```python
from build123d import *

# Parameters (mm, degrees)
SKETCH1_W                = 82
SKETCH1_H                = 150
BOSS_EXTRUDE1_DEPTH      = 10
SKETCH2_W                = 10
SKETCH2_H                = 45
BOSS_EXTRUDE2_DEPTH      = 82
BOSS_EXTRUDE3_DEPTH      = 42
BOSS_EXTRUDE3_DEPTH_BACK = 10
FILLET3_RADIUS           = 26
FILLET3_LENGTH           = 10
FILLET4_RADIUS           = 26
FILLET4_LENGTH           = 10
BOSS_EXTRUDE4_DEPTH      = 10
BOSS_EXTRUDE5_DEPTH      = 10
FILLET5_R                = 15
FILLET6_R                = 15
SKETCH6_R                = 8
SKETCH6_R_2              = 5.5
CUT_EXTRUDE1_DEPTH       = 131.057679512
FILLET7_R                = 3
FILLET8_R                = 3
FILLET9_R                = 3
FILLET10_R               = 3
FILLET11_R               = 2
SKETCH7_R                = 5.5
CUT_EXTRUDE2_DEPTH       = 116.043470045
SKETCH8_W                = 188.706485039
SKETCH8_H                = 108.604028409
CUT_EXTRUDE3_DEPTH       = 126.678160394
SKETCH9_W                = 188.802330386
SKETCH9_H                = 115.284492933
CUT_EXTRUDE4_DEPTH       = 119.718153624
SKETCH10_W               = 24.217021772
SKETCH10_H               = 20.660675918
SKETCH10_W_2             = 13.71733401
SKETCH10_H_2             = 13.378634406
BOSS_EXTRUDE6_DEPTH      = 10


with BuildPart() as part:
    # Sketch1 → Boss-Extrude1 (new body)
    with BuildSketch(Plane(origin=(0, 0, 0), x_dir=(1, 0, 0), z_dir=(0, 1, 0))):
        Rectangle(SKETCH1_W, SKETCH1_H)
    extrude(amount=BOSS_EXTRUDE1_DEPTH)

    # Sketch2 → Boss-Extrude2 (add, through all)
    with BuildSketch(Plane(origin=(41, 0, 0), x_dir=(0, 0, -1), z_dir=(1, 0, 0))):
        with Locations((70, 22.5)):
            Rectangle(SKETCH2_W, SKETCH2_H)
    extrude(amount=-BOSS_EXTRUDE2_DEPTH)

    # Sketch3 → Boss-Extrude3 (add, two sides: drawn at the far end of the back side and taken through both)
    with BuildSketch(Plane.XY.offset(-65).offset(-BOSS_EXTRUDE3_DEPTH_BACK)):
        Polygon((10, 45), (10, 10), (20, 10), (20, 45), (20, 87), (10, 87), align=None)
        Polygon((-10, 45), (-10, 87), (-20, 87), (-20, 45), (-20, 10), (-10, 10), align=None)
    extrude(amount=BOSS_EXTRUDE3_DEPTH + BOSS_EXTRUDE3_DEPTH_BACK)

    # Fillet3: full round fillet: the end face becomes a half cylinder, R = half its width
    fillet3_face = Plane((15, 87, -49), x_dir=(-1, 0, 0), z_dir=(0, 1, 0))  # on the end face: x along it, z out of the body
    fillet3_slab = fillet3_face.offset(-FILLET3_RADIUS / 2) * Box(FILLET3_LENGTH, 2 * FILLET3_RADIUS, FILLET3_RADIUS, mode=Mode.PRIVATE)  # the body's end, R deep
    fillet3_round = Plane((15, 61, -49), x_dir=(0, 1, 0), z_dir=(-1, 0, 0)) * Cylinder(FILLET3_RADIUS, FILLET3_LENGTH, mode=Mode.PRIVATE)  # its axis R under the face
    add(fillet3_slab - fillet3_round, mode=Mode.SUBTRACT)

    # Fillet4: full round fillet: the end face becomes a half cylinder, R = half its width
    fillet4_face = Plane((-15, 87, -49), x_dir=(-1, 0, 0), z_dir=(0, 1, 0))  # on the end face: x along it, z out of the body
    fillet4_slab = fillet4_face.offset(-FILLET4_RADIUS / 2) * Box(FILLET4_LENGTH, 2 * FILLET4_RADIUS, FILLET4_RADIUS, mode=Mode.PRIVATE)  # the body's end, R deep
    fillet4_round = Plane((-15, 61, -49), x_dir=(0, 1, 0), z_dir=(-1, 0, 0)) * Cylinder(FILLET4_RADIUS, FILLET4_LENGTH, mode=Mode.PRIVATE)  # its axis R under the face
    add(fillet4_slab - fillet4_round, mode=Mode.SUBTRACT)

    # Sketch4 → Boss-Extrude4 (add)
    with BuildSketch(Plane(origin=(20, 0, 0), x_dir=(0, 0, -1), z_dir=(1, 0, 0))):
        Polygon((23, 10), (23, 50), (-75, 25), (-75, 10), align=None)
    extrude(amount=-BOSS_EXTRUDE4_DEPTH)

    # Sketch5 → Boss-Extrude5 (add)
    with BuildSketch(Plane.ZY.offset(20)):
        Polygon((-23, 50), (75, 25), (75, 10), (-23, 10), align=None)
    extrude(amount=-BOSS_EXTRUDE5_DEPTH)

    # Fillet5
    fillet5_edges = [part.edges().sort_by_distance(p)[0] for p in [
        (15, 25, 75),
    ]]
    fillet(fillet5_edges, radius=FILLET5_R)

    # Fillet6
    fillet6_edges = [part.edges().sort_by_distance(p)[0] for p in [
        (-15, 25, 75),
    ]]
    fillet(fillet6_edges, radius=FILLET6_R)

    # Sketch6 → Cut-Extrude1 (cut, through all)
    with BuildSketch(Plane(origin=(20, 0, 0), x_dir=(0, 0, -1), z_dir=(1, 0, 0))):
        with Locations((49, 61)):
            Circle(SKETCH6_R)
        with Locations((-60, 17.5)):
            Circle(SKETCH6_R_2)
    extrude(amount=-CUT_EXTRUDE1_DEPTH, mode=Mode.SUBTRACT)

    # Fillet7
    fillet7_edges = [part.edges().sort_by_distance(p)[0] for p in [
        (30.5, 45, -65),
    ]]
    fillet(fillet7_edges, radius=FILLET7_R)

    # Fillet8
    fillet8_edges = [part.edges().sort_by_distance(p)[0] for p in [
        (0, 45, -65),
    ]]
    fillet(fillet8_edges, radius=FILLET8_R)

    # Fillet9
    fillet9_edges = [part.edges().sort_by_distance(p)[0] for p in [
        (-30.5, 45, -65),
    ]]
    fillet(fillet9_edges, radius=FILLET9_R)

    # Fillet10
    fillet10_edges = [part.edges().sort_by_distance(p)[0] for p in [
        (30.5, 10, -65),
        (0, 10, -65),
        (-30.5, 10, -65),
    ]]
    fillet(fillet10_edges, radius=FILLET10_R)

    # Fillet11
    fillet11_edges = [part.edges().sort_by_distance(p)[0] for p in [
        (15, 50, -23),
        (-15, 50, -23),
    ]]
    fillet(fillet11_edges, radius=FILLET11_R)

    # Sketch7 → Cut-Extrude2 (cut, through all)
    with BuildSketch(Plane(origin=(0, 10, 0), x_dir=(1, 0, 0), z_dir=(0, 1, 0))):
        with Locations(Location((31.5, 45, 0), (0, 0, 270))):
            Circle(SKETCH7_R)
        with Locations(Location((31.5, -15, 0), (0, 0, 270))):
            Circle(SKETCH7_R)
        with Locations(Location((-31.5, -15, 0), (0, 0, 90))):
            Circle(SKETCH7_R)
        with Locations(Location((-31.5, 45, 0), (0, 0, 90))):
            Circle(SKETCH7_R)
    extrude(amount=-CUT_EXTRUDE2_DEPTH, mode=Mode.SUBTRACT)

    # Sketch8 → Cut-Extrude3 (cut, through all)
    with BuildSketch(Plane.ZY.offset(-10)):
        with Locations((0.093142392, 45.704427175)):
            Rectangle(SKETCH8_W, SKETCH8_H)
    extrude(amount=-CUT_EXTRUDE3_DEPTH, mode=Mode.SUBTRACT)

    # Sketch9 → Cut-Extrude4 (cut, through all)
    with BuildSketch(Plane.ZY.offset(20)):
        with Locations((2.13095181, 34.866066892)):
            Rectangle(SKETCH9_W, SKETCH9_H)
    extrude(amount=CUT_EXTRUDE4_DEPTH, mode=Mode.SUBTRACT)

    # Sketch10 → Boss-Extrude6 (add)
    with BuildSketch(Plane.ZY.offset(20)):
        with Locations((-48.857418051, 60.43498026)):
            Rectangle(SKETCH10_W, SKETCH10_H)
        with Locations((60.54255443, 16.996755893)):
            Rectangle(SKETCH10_W_2, SKETCH10_H_2)
    extrude(amount=-BOSS_EXTRUDE6_DEPTH)


solid = part.part
```
Geometry: final body of the model. Coordinates: model frame, mm. A direction names the side the tool comes from. Coordinates: 2 decimals unless noted, no trailing zeros. Order: outer loops, then holes, each group sorted by start corner. A loop starts at its lowest first (then second) coordinate and runs counter-clockwise, first axis right, second up. Notation, with made-up numbers: M -14.5,43.5 L 43.5,43.5 A31 cw 43.5,75.5 Z; hole C 73.25,55 d8. An arc over 180 degrees is marked long. Answer in a Markdown table with one row per item. Add a question column.
Q1. Line query: L1, parallel to Y at x = -0.75, z = 28; L2, parallel to Z at x = 5.5, y = 39; L3, parallel to X at y = 15, z = -44. Output: solid intervals per line, ascending.
Q2. Reachability of faces 4 (the flat face through (-5, 0, -1)), 5 (the cylindrical face through (-0.14, 44.14, -65.9)), 6 (the flat face through (0, 45, -71)) from +Z, -Z, +X, -X, +Y, -Y: full face, straight path, thin tool, end or side. Return the list, or none.
Q3. Section query D-D on z = 66. Return the cut outline in (x, y), and give its area (3 significant figures).
Q4. Section query B-B on z = -49. Return the cut outline in (x, y), and give its area (3 significant figures).
Q5. Mould query, pull axis X, two halves, no side actions, for faces 1 (the flat face through (10, 9, -17)), 2 (the flat face through (-20, 34, -16)), 3 (the flat face through (-15, 56, -23)). Classes: released by +X, released by -X, zero draft, split by the parting line, or undercut.
Q6. Section query A-A on x = 5.5. Return the cut outline in (y, z), and give its area (3 significant figures).
Q7. Section query C-C on y = 47.5. Return the cut outline in (x, z), and give its area (3 significant figures).
Q8. Contact query for flat-ended pins moving along their axis: P1, Ø3, axis at x = -1, z = 27, coming from the -Y side; P2, Ø4.5, axis at x = -17, y = 57, coming from the +Z side; P3, Ø3, axis at y = 27.5, z = 54.5, coming from the +X side; P4, Ø12, axis at x = -15.5, y = 24, coming from the +Z side. Output: stop coordinate, or through.
Completed:
| question | item | result |
|---|---|---|
| 1 | L1 | y = 0 to 10 |
| 1 | L2 | z = -75 to -65 |
| 1 | L3 | x = -20 to -10 |
| 2 | face 4 | +Z, -Z, +X, -X, -Y |
| 2 | face 5 | +Z, +X, +Y |
| 2 | face 6 | +Z, -Z, +X, +Y |
| 3 | outline | M -20,0 L 10,0 L 10,10 L -10,10 L -10,27.09 L -20,27.09 Z |
| 3 | area | 471 mm2 |
| 4 | outline | M -20,0 L 10,0 L 10,10 L -10,10 L -10,87 L -20,87 Z |
| 4 | area | 1,070 mm2 |
| 5 | face 1 | released by +X |
| 5 | face 2 | released by -X |
| 5 | face 3 | zero draft |
| 6 | outline | M 0,-75 L 45,-75 L 45,-68 A3 ccw 42,-65 L 13,-65 A3 cw 10,-62 L 10,75 L 0,75 Z |
| 6 | area | 1,850 mm2 |
| 7 | outline | M -20,-75 L -10,-75 L -10,-13.2 L -20,-13.2 Z |
| 7 | area | 618 mm2 |
| 8 | P1 | stops at y = 0 |
| 8 | P2 | stops at z = -23 |
| 8 | P3 | stops at x = -10 |
| 8 | P4 | stops at z = 74.26 |
